Job drawing, mm, ordinate dimensions from the low corner. One solid piece. A direction names the side the tool comes from. Round coordinates to 2 decimals unless told otherwise and drop trailing zeros. Loops run counter-clockwise (first coordinate to the right, second up) from the corner with the lowest first, then second, coordinate; pieces in that order, holes last. Notation, with made-up numbers: M 41,83.5 L 80,83.5 A26 ccw 80,100.5 Z; hole C 33.5,65.25 d2. An arc over 180 degrees is marked long. Use one line per item in the form item = value.
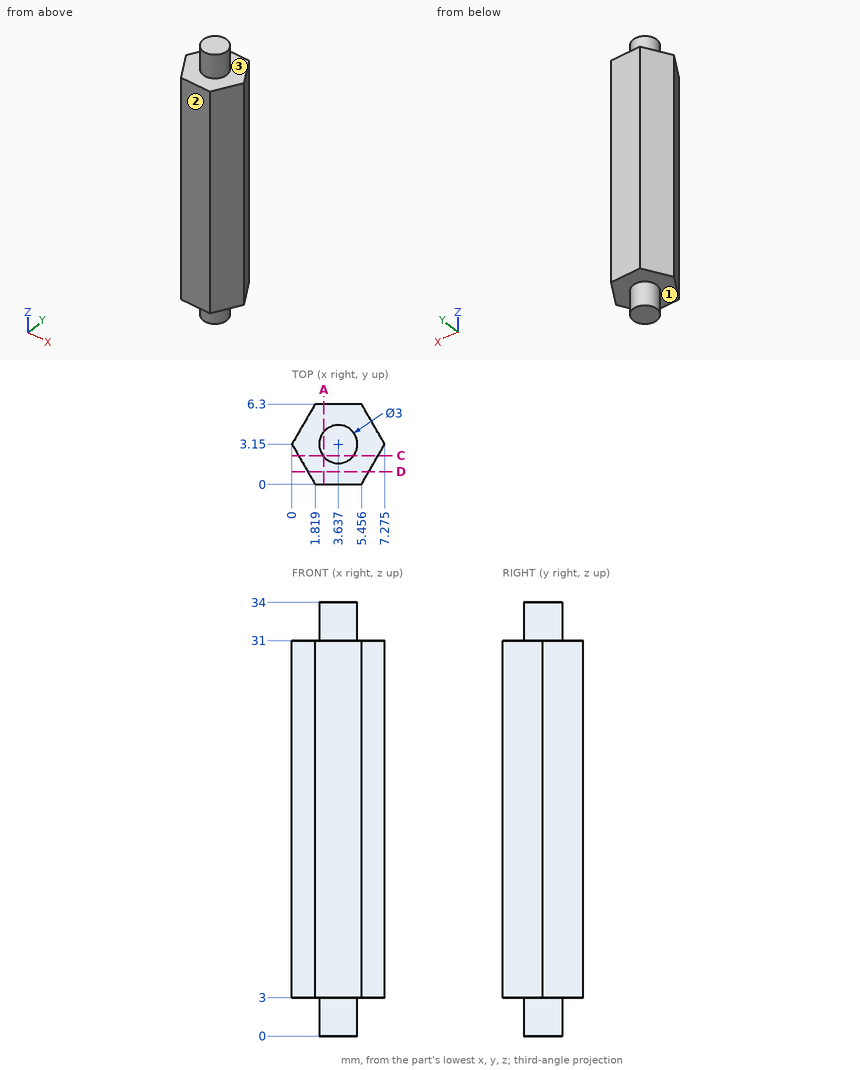
1. Cut at A-A on x = 2.5. Write the cut outline in (y, z).
Completed:
outline = M 0,3 L 2.17,3 L 2.17,0 L 4.13,0 L 4.13,3 L 6.3,3 L 6.3,31 L 4.13,31 L 4.13,34 L 2.17,34 L 2.17,31 L 0,31 Z
2. Tool access for the marked faces 1, 2 and 3: list every direction of +Z, -Z, +X, -X, +Y, -Y with a clear straight run to the whole face (end or side of a thin tool).
Completed:
face_1 = -Z
face_2 = +Z, -Z, +X, -X, -Y
face_3 = +Z
3. Cut at D-D on y = 1. Write the cut outline in (x, z).
Completed:
outline = M 1.24,3 L 6.03,3 L 6.03,31 L 1.24,31 Z
4. Cut at C-C on y = 2.25. Write the cut outline in (x, z) (1 decimal).
Completed:
outline = M 0.5,3 L 2.4,3 L 2.4,0 L 4.8,0 L 4.8,3 L 6.8,3 L 6.8,31 L 4.8,31 L 4.8,34 L 2.4,34 L 2.4,31 L 0.5,31 Z
5. Probe line 1 along Z through (x, y) = (2, 3.75); line 2 along Y through (x, z) = (3.5, 32); line 3 along X through (y, z) = (2, 14) (1 decimal). List the from-to ranges inside material, lowest first. Write a range as from..to.
Completed:
line_1 = 3..31
line_2 = 1.66..4.64
line_3 = 0.7..6.6
